The model under review builds one solid part; all positions refer to its coordinate system, in mm. A direction names the side the tool comes from. Round coordinates to 2 decimals unless told otherwise and drop trailing zeros. Loops run counter-clockwise (first coordinate to the right, second up) from the corner with the lowest first, then second, coordinate; pieces in that order, holes last. Notation, with made-up numbers: (20.25, 66) -> (36.25, 66) arc R15 cw to (36.25, 74) -> close; hole circle Ø7 at (66, -24). An arc over 180 degrees is marked (long way). Use CSV: the item, a comma, the result in double quotes. Start each with the question number.
```python
from build123d import *

# Parameters (mm, degrees)
SKETCH1_W           = 168.402
SKETCH1_H           = 41.275
BOSS_EXTRUDE1_DEPTH = 6.35
CUT_EXTRUDE1_DEPTH  = 87.925469842
CUT_EXTRUDE2_DEPTH  = 87.925469842


with BuildPart() as part:
    # Sketch1 → Boss-Extrude1 (new body)
    with BuildSketch(Plane.XY):
        Rectangle(SKETCH1_W, SKETCH1_H)
    extrude(amount=BOSS_EXTRUDE1_DEPTH)

    # Sketch2 → Cut-Extrude1 (cut, through all)
    with BuildSketch(Plane.XY.offset(6.35)):
        with BuildLine():
            Line((63.5, -14.351), (-63.5, -14.351))
            ThreePointArc((-63.5, -14.351), (-77.851, 0), (-63.5, 14.351))
            Line((-63.5, 14.351), (63.5, 14.351))
            ThreePointArc((63.5, 14.351), (77.851, 0), (63.5, -14.351))
        make_face()
    extrude(amount=-CUT_EXTRUDE1_DEPTH, mode=Mode.SUBTRACT)

    # Sketch5 → Cut-Extrude2 (cut, through all)
    with BuildSketch(Plane.XY.offset(6.35)):
        with BuildLine():
            ThreePointArc((-84.201, -7.7e-08), (-78.699849051, 14.053326646), (-65.120183554, 20.6375))
            Line((-65.120183554, 20.6375), (-84.201, 20.6375))
            Line((-84.201, 20.6375), (-84.201, -7.7e-08))
        make_face()
        with BuildLine():
            ThreePointArc((-65.120183554, -20.6375), (-78.699848999, -14.053326703), (-84.201, -7.7e-08))
            Line((-84.201, -7.7e-08), (-84.201, -20.6375))
            Line((-84.201, -20.6375), (-65.120183554, -20.6375))
        make_face()
        with BuildLine():
            Line((84.201, 20.6375), (65.120183554, 20.6375))
            ThreePointArc((65.120183554, 20.6375), (78.699849025, 14.053326674), (84.201, 0))
            Line((84.201, 0), (84.201, 20.6375))
        make_face()
        with BuildLine():
            Line((84.201, -20.6375), (84.201, 0))
            ThreePointArc((84.201, 0), (78.699849025, -14.053326674), (65.120183554, -20.6375))
            Line((65.120183554, -20.6375), (84.201, -20.6375))
        make_face()
    extrude(amount=-CUT_EXTRUDE2_DEPTH, mode=Mode.SUBTRACT)


solid = part.part
```
1. Take a section at A-A, the plane x = 4. Give the boundary of the cut face in (y, z), then the cut area to 3 significant figures.
2. Take a section at B-B, the plane z = 1.5. Give the boundary of the cut face in (x, y), then the cut area to 3 significant figures.
3. The part is to be moulded in two halves that separate along X. For faces 1 (the face through (-1, 14.351, 3)), 2 (the face through (0, -17, 0)), say which applies: pulls with the +X half, pulls with the -X half, needs draft (parallel to the pull), parting line crosses it, or undercut.
4. For faces 3 (the face through (-1, 20.638, 3)), 4 (the face through (1, -14.351, 3)), list the 3-axis set-ups (+Z, -Z, +X, -X, +Y, -Y) from which the entire face can be reached by the end or side of a thin tool; tool diameter is ignored.
5. For line 1 along Y through (x, z) = (-7, 5.75); line 2 along X through (y, z) = (-3, 4.5); line 3 along X through (y, z) = (-11, 4.5), list the stretches that pass through material, from the lowest coordinate up. Write a range as from..to.
6. Take a section at C-C, the plane y = -4. Give the boundary of the cut face in (x, z), then the cut area to 3 significant figures.
Results:
1,outline,"(-20.64, 0) -> (-14.35, 0) -> (-14.35, 6.35) -> (-20.64, 6.35) -> close; (14.35, 0) -> (20.64, 0) -> (20.64, 6.35) -> (14.35, 6.35) -> close"
1,area,"79.8 mm²"
2,outline,"(-65.12, -20.64) -> (65.12, -20.64) arc R20.7 ccw to (65.12, 20.64) -> (-65.12, 20.64) arc R20.7 ccw to start; hole (-63.5, -14.35) -> (63.5, -14.35) arc R14.35 ccw to (63.5, 14.35) -> (-63.5, 14.35) arc R14.35 ccw to start"
2,area,"2,300 mm²"
3,face 1,"undercut"
3,face 2,"needs draft"
4,face 3,"+Z, -Z, +X, -X, +Y"
4,face 4,"+Z, -Z"
5,line 1,"-20.64..-14.35, 14.35..20.64"
5,line 2,"-83.98..-77.53, 77.53..83.98"
5,line 3,"-81.04..-72.72, 72.72..81.04"
6,outline,"(-83.81, 0) -> (-77.28, 0) -> (-77.28, 6.35) -> (-83.81, 6.35) -> close; (77.28, 0) -> (83.81, 0) -> (83.81, 6.35) -> (77.28, 6.35) -> close"
6,area,"82.9 mm²"
